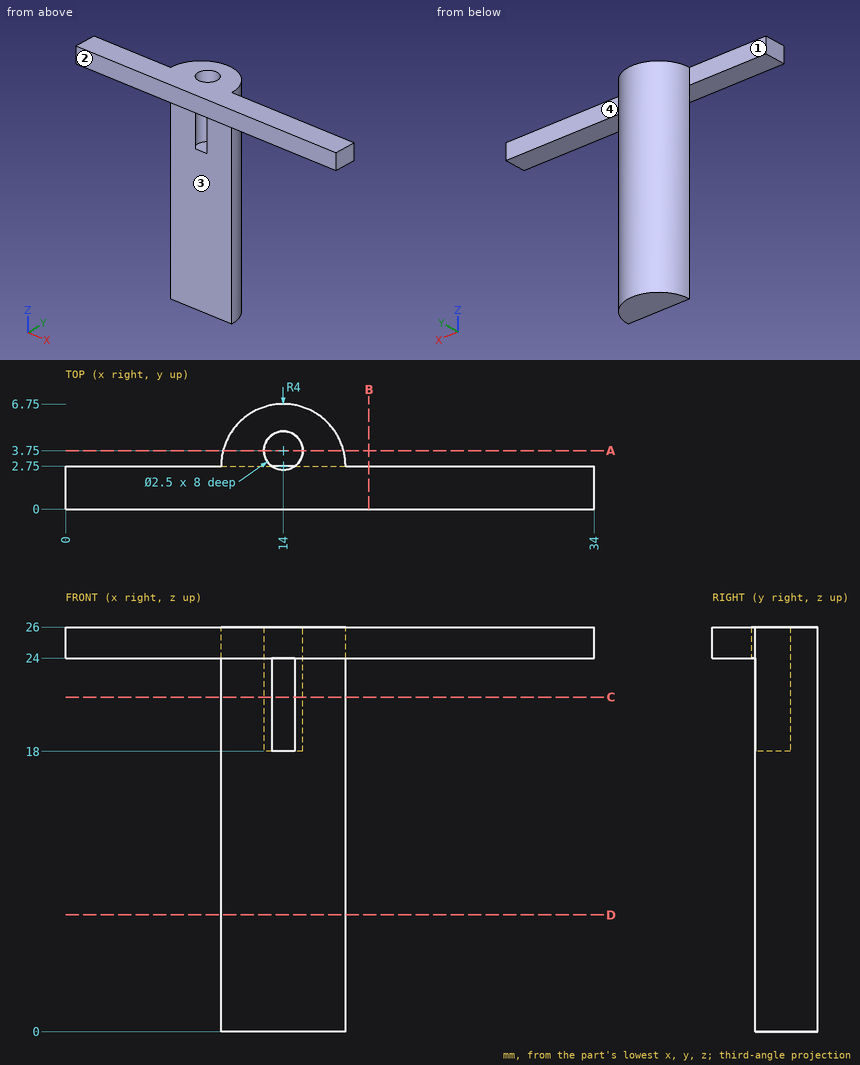
Print and shaded views of the part. All mm, measured from the part's lowest x, y and z. A direction names the side the tool comes from. Give positions to 0.01 mm unless a question says otherwise; leave off trailing zeros. Loops run counter-clockwise (first coordinate to the right, second up) from the corner with the lowest first, then second, coordinate; pieces in that order, holes last.
1) Saw through at C-C (z = 21.5). Write the cut outline in (x, y).
2) Saw through at B-B (x = 19.5). Write the cut outline in (y, z), plus the area to 3 significant figures.
3) Saw through at D-D (z = 7.5). Write the cut outline in (x, y), plus the area to 3 significant figures.
4) Wall check: line 1 (Z direction, x = 15, y = 2.25); line 2 (Y direction, x = 14, z = 21.75); line 3 (X direction, y = 3.75, z = 20.75). Give the ranges that are in metal, low to high.
5) Flat gauge pins, fed straight in: pin 1 Ø4 at (y, z) = (3, 17.5) entering from +X; pin 2 Ø2 at (x, y) = (19.5, 2) entering from -Z; pin 3 Ø1.5 at (y, z) = (5, 3.5) entering from +X; pin 4 Ø2 at (x, y) = (14, 3.75) entering from -Z. Where does each tip first touch, or does it go through?
6) Saw through at A-A (y = 3.75). Write the cut outline in (x, z).
7) Tool access for the marked faces 1, 2, 3 and 4: list every direction of +Z, -Z, +X, -X, +Y, -Y with a clear straight run to the whole face (end or side of a thin tool).
Answer block:
1. outline: (10, 2.75) - (13.25, 2.75) arc R1.25 cw (long way) to (14.75, 2.75) - (18, 2.75) arc R4 ccw to start
2. outline: (0, 24) - (2.75, 24) - (2.75, 26) - (0, 26) - close
2. area: 5.50 mm2
3. outline: (10, 2.75) - (18, 2.75) arc R4 ccw to start
3. area: 25.1 mm2
4. line 1: z = 24 to 26
4. line 2: y = 5 to 6.75
4. line 3: x = 10.13 to 12.75, 15.25 to 17.87
5. pin 1: stops at x = 18
5. pin 2: stops at z = 24
5. pin 3: stops at x = 17.71
5. pin 4: stops at z = 0
6. outline: (10.13, 0) - (17.87, 0) - (17.87, 26) - (15.25, 26) - (15.25, 18) - (12.75, 18) - (12.75, 26) - (10.13, 26) - close
7. face 1: +Z, -Z, -X, +Y
7. face 2: +Z, -Z, +X, -X, -Y
7. face 3: -Z, +X, -X, -Y
7. face 4: +Z, -Z, +X, +Y
